The model under review builds one solid part; all positions refer to its coordinate system, in mm. A direction names the side the tool comes from. Give positions to 0.01 mm unless a question says otherwise; leave off trailing zeros. Loops run counter-clockwise (first coordinate to the right, second up) from the corner with the lowest first, then second, coordinate; pieces in that order, holes last. Notation, with made-up numbers: M 56.25,-17.75 L 107.25,-17.75 A29 cw 107.25,16.25 Z; hole C 77.5,30 d8. An arc over 180 degrees is marked long. One line per item, written item: value. Start each with the question number.
Q1. For pin 1 (1.6 mm diameter, centred on x = 2, z = 0, fed in from +Y); pin 2 (0.9 mm diameter, centred on x = 9.5, y = 2, fed in from +Z); pin 3 (1.5 mm diameter, centred on x = 3, z = 1.5, fed in from -Y), all flat-tipped, find the tip position at first contact; note any pin that passes through.
Q2. For faces 1 (the face through (0, 0, 0)), 2 (the face through (24.5, -1.6, 0)), 3 (the face through (11, 2, 1.4)), 4 (the face through (22, 0.8, 1.4)), list the 3-axis set-ups (+Z, -Z, +X, -X, +Y, -Y) from which the entire face can be reached by the end or side of a thin tool; tool diameter is ignored.
Q3. We need section A-A on z = 0. Write out the cut boundary in (x, y), plus the area to 3 significant figures.
Q4. To check wall thickness, follow line 1 along Z through (x, y) = (2, 2.55); line 2 along X through (y, z) = (2.55, 0); line 3 along Z through (x, y) = (21, 1.75). State the ranges of each line that lie inside material, in increasing order. Write a range as from..to.
Q5. We need section D-D on x = 24.75. Write out the cut boundary in (y, z).
Q6. We need section C-C on y = -1.1. Write out the cut boundary in (x, z).
Q7. We need section B-B on x = 2. Write out the cut boundary in (y, z), plus the area to 3 significant figures.
Q8. Mouldability with a two-part tool opening along Z and no side actions: class faces 5 (the face through (11, 2.6, 0)), 6 (the face through (11, 2, -1.4)), 7 (the face through (2, 2.5, 0)), 8 (the face through (24.5, 1.6, 0)) as released by +Z, released by -Z, zero draft, split by the parting line, or undercut.
Autodesk Inventor part; units mm, degrees
ref_plane "SW_SM_XY" through (0, 0, 0) normal (1, 0, 0) x (0, 0, -1)
ref_plane "SW_SM_YZ" through (0, 0, 0) normal (0, 0, -1) x (0, 1, 0)
ref_plane "SW_SM_ZX" through (0, 0, 0) normal (0, 1, 0) x (1, 0, 0)
sketch "Sketch_12" plane through (0, 0, 0) normal (1, 0, 0) x (0, 1, 0)
  arc A0 (1.4283, 1.4) -> (1.4283, -1.4) centre (0, 0) ccw
  line L0 (1.4283, -1.4) -> (2.6, -1.4)
  line L1 (2.6, -1.4) -> (2.6, 1.4)
  line L2 (2.6, 1.4) -> (1.4283, 1.4)
extrude "Extrusion1" add sketch "Sketch_12" along normal blind 22
sketch "Sketch_13" plane through (0, 0, 0) normal (1, 0, 0) x (0, 1, 0)
  line L0 (0.25, 1.35) -> (-0.25, 1.35)
  arc A0 (-0.25, 1.35) -> (-0.25, -1.35) centre (-0.25, 0) ccw
  line L1 (-0.25, -1.35) -> (0.25, -1.35)
  arc A1 (0.25, -1.35) -> (0.25, 1.35) centre (0.25, 0) ccw
extrude "Extrusion2" add sketch "Sketch_13" along normal blind 27
sketch "Sketch3" plane through (0, 2.6, 1.4) normal (0, 1, 0) x (1, 0, 0)
  point P0 (2, 1.4)
hole "Hole1" at (2, 2.6, 0) direction (0, -1, 0) diameter 2 depth 0.1
ref_plane "SW_SM_XY" through (0, 0, 0) normal (1, 0, 0) x (0, 0, -1)
ref_plane "SW_SM_YZ" through (0, 0, 0) normal (0, 0, -1) x (0, 1, 0)
ref_plane "SW_SM_ZX" through (0, 0, 0) normal (0, 1, 0) x (1, 0, 0)
properties part number "CP96-M9P_SW" material "Stainless Steel, Polished"
Solved:
1. pin 1: y = 2.5
1. pin 2: z = 1.4
1. pin 3: y = -1.85
2. face 1: +Z, -Z, -X, +Y, -Y
2. face 2: +X, -Y
2. face 3: +Z, +X, -X, +Y
2. face 4: +X
3. outline: M 0,-2 L 22,-2 L 22,-1.6 L 27,-1.6 L 27,1.6 L 22,1.6 L 22,2.6 L 3,2.6 L 3,2.5 L 1,2.5 L 1,2.6 L 0,2.6 Z
3. area: 117 mm2
4. line 1: -1.4..-1, 1..1.4
4. line 2: 0..1, 3..22
4. line 3: -1.4..1.4
5. outline: M -0.25,-1.35 L 0.25,-1.35 A1.35 ccw 0.25,1.35 L -0.25,1.35 A1.35 ccw Z
6. outline: M 0,-1.67 L 22,-1.67 L 22,-1.05 L 27,-1.05 L 27,1.05 L 22,1.05 L 22,1.67 L 0,1.67 Z
7. outline: M 1.43,-1.4 L 2.6,-1.4 L 2.6,-1 L 2.5,-1 L 2.5,1 L 2.6,1 L 2.6,1.4 L 1.43,1.4 A2 ccw long Z
7. area: 14.5 mm2
8. face 5: zero draft
8. face 6: released by -Z
8. face 7: undercut
8. face 8: split by the parting line
